from build123d import *

# Parameters (mm, degrees)
SKETCH_R        = 54
SKETCH_R_2      = 32.5
SKETCH_R_3      = 2.5
PAD_DEPTH       = 3
SKETCH002_R     = 42
SKETCH002_R_2   = 37.5
PAD002_DEPTH    = 19.5
SKETCH003_R     = 37.5
SKETCH003_R_2   = 32.5
PAD003_DEPTH    = 7.5
CHAMFER_SIZE    = 1
CHAMFER001_SIZE = 1


with BuildPart() as part:
    # Sketch → Pad (new body)
    with BuildSketch(Plane.XY):
        Circle(SKETCH_R)
        Circle(SKETCH_R_2, mode=Mode.SUBTRACT)
        with Locations((0, 49)):
            Circle(SKETCH_R_3, mode=Mode.SUBTRACT)
        with Locations((48.25558, 8.508761)):
            Circle(SKETCH_R_3, mode=Mode.SUBTRACT)
        with Locations((42.435245, -24.5)):
            Circle(SKETCH_R_3, mode=Mode.SUBTRACT)
        with Locations((16.758987, -46.044938)):
            Circle(SKETCH_R_3, mode=Mode.SUBTRACT)
        with Locations((-16.758987, -46.044938)):
            Circle(SKETCH_R_3, mode=Mode.SUBTRACT)
        with Locations((-42.435245, -24.5)):
            Circle(SKETCH_R_3, mode=Mode.SUBTRACT)
        with Locations((-48.25558, 8.508761)):
            Circle(SKETCH_R_3, mode=Mode.SUBTRACT)
        with Locations((-31.496593, 37.536178)):
            Circle(SKETCH_R_3, mode=Mode.SUBTRACT)
        with Locations((31.496593, 37.536178)):
            Circle(SKETCH_R_3, mode=Mode.SUBTRACT)
    extrude(amount=PAD_DEPTH)

    # Sketch002 → Pad002 (join)
    with BuildSketch(Plane.XY.offset(3)):
        Circle(SKETCH002_R)
        Circle(SKETCH002_R_2, mode=Mode.SUBTRACT)
    extrude(amount=PAD002_DEPTH)

    # Sketch003 (on Face15 of Pad002) → Pad003 (join)
    with BuildSketch(Plane.XY.offset(3)):
        Circle(SKETCH003_R)
        Circle(SKETCH003_R_2, mode=Mode.SUBTRACT)
    extrude(amount=PAD003_DEPTH)

    # Chamfer
    chamfer_edges = [part.edges().sort_by_distance(p)[0] for p in [
        (-37.5, 0, 22.5),
    ]]
    chamfer(chamfer_edges, length=CHAMFER_SIZE)

    # Chamfer001
    chamfer001_edges = [part.edges().sort_by_distance(p)[0] for p in [
        (-42, 0, 22.5),
    ]]
    chamfer(chamfer001_edges, length=CHAMFER001_SIZE)


solid = part.part
Source: CAD feature listing. Evaluate the final solid. Frame: model axes, mm. A direction names the side the tool comes from. Give positions to 0.01 mm unless a question says otherwise; leave off trailing zeros. Loops run counter-clockwise (first coordinate to the right, second up) from the corner with the lowest first, then second, coordinate; pieces in that order, holes last. Notation, with made-up numbers: (7.5, 82.25) -> (28.5, 82.25) arc R10 ccw to (28.5, 95.25) -> close; hole circle Ø2 at (-5, -5.75). An arc over 180 degrees is marked (long way). Use a Markdown table: item, result. Add a question column.
1) Line query: line 1 along Y through (x, z) = (0, 1.3); line 2 along Y through (x, z) = (0, 17.75); line 3 along Z through (x, y) = (-39.5, 33). Output: solid intervals per line, ascending. Write a range as [from, to].
2) Section query B-B, the plane x = 0. Return the cut outline in (y, z).
3) Section query D-D, the plane y = 49. Return the cut outline in (x, z), then the cut area to 3 significant figures.
4) Reachability of faces 1 (the face through (23.2, -23.2, 0)), 2 (the face through (16, -40, 3)) from +Z, -Z, +X, -X, +Y, -Y: full face, straight path, thin tool, end or side. Return the list, or none.
5) First-contact query: pin 1 (4 mm diameter, centred on y = 35.5, z = 10.5, fed in from -X); pin 2 (10 mm diameter, centred on x = 2, z = 17.5, fed in from -Y); pin 3 (1 mm diameter, centred on x = -35.5, z = 10.5, fed in from +Y). Flat tips, straight axial feed; report the tip coordinate or a pass-through.
6) Pull-direction query (X, two-part tool) for faces 3 (the face through (-37, -12, 22.5)), 4 (the face through (-29.112, 38.287, 1.479)), 5 (the face through (40.06, 12.62, 12.12)); classes: +X half, -X half, draft (parallel to the pull), parting line (faces both ways), or undercut.
7) Section query C-C, the plane z = 13.75. Return the cut outline in (x, y).
8) Section query A-A, the plane y = 0. Return the cut outline in (x, z), then the cut area to 4 significant figures.
Numbers:
| question | item | result |
|---|---|---|
| 1 | line 1 | y = [-54, -32.5], [32.5, 46.5], [51.5, 54] |
| 1 | line 2 | y = [-42, -37.5], [37.5, 42] |
| 1 | line 3 | z = [0, 3] |
| 2 | outline | (-54, 0) -> (-32.5, 0) -> (-32.5, 10.5) -> (-37.5, 10.5) -> (-37.5, 21.5) -> (-38.5, 22.5) -> (-41, 22.5) -> (-42, 21.5) -> (-42, 3) -> (-54, 3) -> close; (32.5, 0) -> (46.5, 0) -> (46.5, 3) -> (42, 3) -> (42, 21.5) -> (41, 22.5) -> (38.5, 22.5) -> (37.5, 21.5) -> (37.5, 10.5) -> (32.5, 10.5) -> close; (51.5, 0) -> (54, 0) -> (54, 3) -> (51.5, 3) -> close |
| 3 | outline | (-22.69, 0) -> (-2.5, 0) -> (-2.5, 3) -> (-22.69, 3) -> close; (2.5, 0) -> (22.69, 0) -> (22.69, 3) -> (2.5, 3) -> close |
| 3 | area | 121 mm2 |
| 4 | face 1 | -Z, +X, -X, +Y, -Y |
| 4 | face 2 | +Z |
| 5 | pin 1 | stops at x = -25.33 |
| 5 | pin 2 | stops at y = -42 |
| 5 | pin 3 | stops at y = 23.22 |
| 6 | face 3 | draft |
| 6 | face 4 | undercut |
| 6 | face 5 | parting line |
| 7 | outline | circle Ø84 at (0, 0); hole circle Ø75 at (0, 0) |
| 8 | outline | (-54, 0) -> (-32.5, 0) -> (-32.5, 10.5) -> (-37.5, 10.5) -> (-37.5, 21.5) -> (-38.5, 22.5) -> (-41, 22.5) -> (-42, 21.5) -> (-42, 3) -> (-54, 3) -> close; (32.5, 0) -> (54, 0) -> (54, 3) -> (42, 3) -> (42, 21.5) -> (41, 22.5) -> (38.5, 22.5) -> (37.5, 21.5) -> (37.5, 10.5) -> (32.5, 10.5) -> close |
| 8 | area | 377.5 mm2 |
